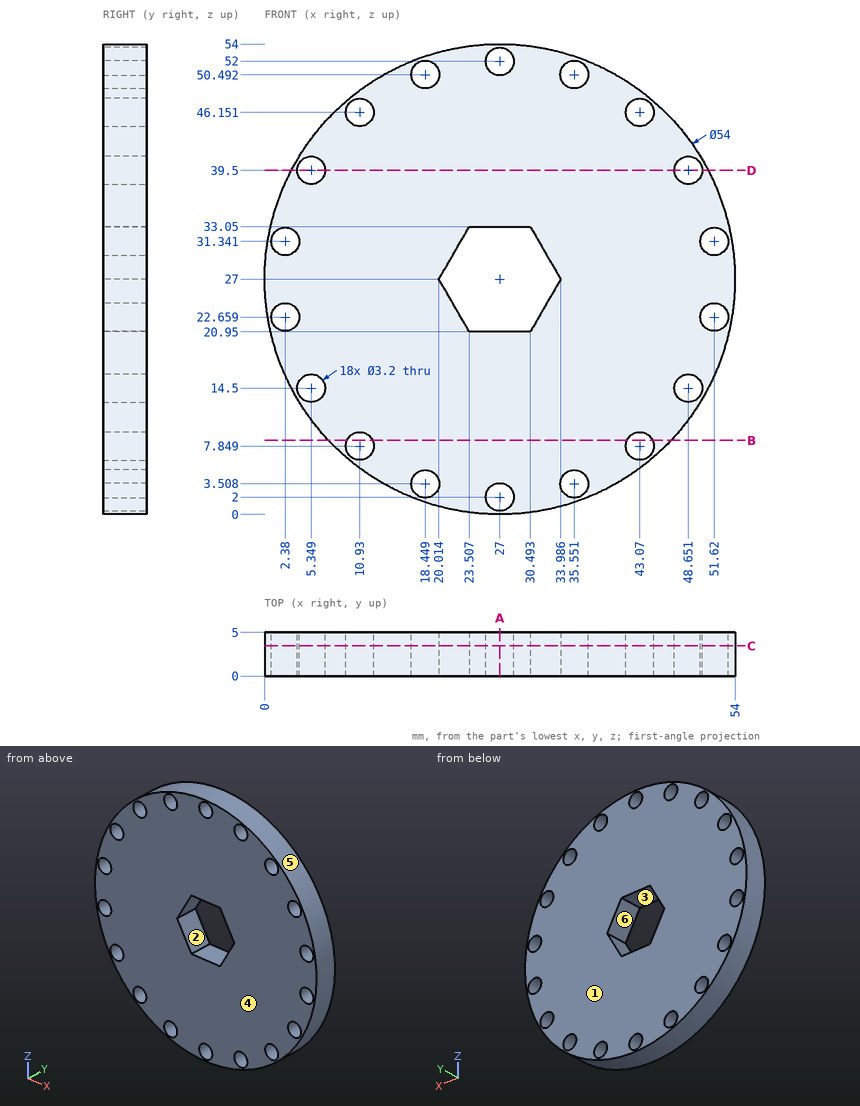
Input: dimensioned drawing with shaded views. Units: mm. Origin: part minimum x, y, z. A direction names the side the tool comes from. Give positions to 0.01 mm unless a question says otherwise; leave off trailing zeros. Order: outer loops, then holes, each group sorted by start corner. A loop starts at its lowest first (then second) coordinate and runs counter-clockwise, first axis right, second up. Notation, with made-up numbers: (-28, 38) -> (-23, 38) arc R21 ccw to (-23, 67) -> close; hole circle Ø6 at (-21, 33). An arc over 180 degrees is marked (long way). Answer as a JSON object with one key per item and string values.
Q1. Access query for the marked faces 1 and 2. Directions: +Z, -Z, +X, -X, +Y, -Y. A direction counts if a zero-diameter tool reaches every point of the face in a straight line with its end or side. Return the directions, or none.
Entries:
{"face 1": "+Z, -Z, +X, -X, +Y", "face 2": "+Y, -Y"}
Q2. Section B-B (z = 8.5). Output: boundary loops of the cut face in (x, y) (1 decimal).
Entries:
{"outline": "(7.3, 0) -> (9.5, 0) -> (9.5, 5) -> (7.3, 5) -> close; (12.4, 0) -> (41.6, 0) -> (41.6, 5) -> (12.4, 5) -> close; (44.5, 0) -> (46.7, 0) -> (46.7, 5) -> (44.5, 5) -> close"}
Q3. Section C-C (y = 3.45). State how many separate pieces and enclosed holes the cut face has, plus the area to 3 significant figures.
Entries:
{"separate pieces": "1", "enclosed holes": "19", "area": "2,020 mm^2"}
Q4. Draft query along Z for the marked faces 3, 4, 5 and 6. Return one class per face: released by +Z, released by -Z, zero draft, split by the parting line, or undercut.
Entries:
{"face 3": "undercut", "face 4": "zero draft", "face 5": "split by the parting line", "face 6": "undercut"}
Q5. Section A-A (x = 27). Output: boundary loops of the cut face in (y, z).
Entries:
{"outline": "(0, 0) -> (5, 0) -> (5, 0.4) -> (0, 0.4) -> close; (0, 3.6) -> (5, 3.6) -> (5, 20.95) -> (0, 20.95) -> close; (0, 33.05) -> (5, 33.05) -> (5, 50.4) -> (0, 50.4) -> close; (0, 53.6) -> (5, 53.6) -> (5, 54) -> (0, 54) -> close"}
Q6. Material intervals for probe 1 along X at (y, z) = (3.9, 39.5); probe 2 along Z at (x, y) = (28, 3); probe 3 along Z at (x, y) = (47.5, 0.5) (1 decimal), sorted ascending.
Entries:
{"probe 1": "x = 3.07 to 3.75, 6.95 to 47.05, 50.25 to 50.93", "probe 2": "z = 0.02 to 0.75, 3.25 to 20.95, 33.05 to 50.75, 53.25 to 53.98", "probe 3": "z = 9.4 to 13.4, 15.6 to 38.4, 40.6 to 44.6"}
Q7. Section D-D (z = 39.5). Output: boundary loops of the cut face in (x, y).
Entries:
{"outline": "(3.07, 0) -> (3.75, 0) -> (3.75, 5) -> (3.07, 5) -> close; (6.95, 0) -> (47.05, 0) -> (47.05, 5) -> (6.95, 5) -> close; (50.25, 0) -> (50.93, 0) -> (50.93, 5) -> (50.25, 5) -> close"}
Q8. First-contact query: pin 1 (4 mm diameter, centred on x = 48.65, z = 39.5, fed in from -Y); pin 2 (3 mm diameter, centred on y = 2.5, z = 45, fed in from +X); pin 3 (2 mm diameter, centred on x = 25, y = 4.5, fed in from -Z); pin 4 (2 mm diameter, centred on x = 37.5, y = 3.5, fed in from +Z). Flat tips, straight axial feed; report the tip coordinate or a pass-through.
Entries:
{"pin 1": "stops at y = 0", "pin 2": "stops at x = 48.37", "pin 3": "stops at z = 0.02", "pin 4": "stops at z = 52.27"}
